Read the model definition and answer for the solid it produces. Units are mm, in the model's axes. Face numbers are marked on the shaded views. A direction names the side the tool comes from. Give positions to 0.01 mm unless a question says otherwise; leave off trailing zeros. Order: outer loops, then holes, each group sorted by start corner. A loop starts at its lowest first (then second) coordinate and runs counter-clockwise, first axis right, second up.
Item 1: A cutting plane is placed at C-C (x = -8.5). Write down the section's boundary in (y, z), plus the area to 3 significant figures.
Item 2: A cutting plane is placed at D-D (y = 1.5). Write down the section's boundary in (x, z).
Item 3: Find the intervals of material crossed by line 1 along Y through (x, z) = (-8.5, -0.5); line 2 along Y through (x, z) = (13, -0.25); line 3 along Z through (x, y) = (2, 7.5) (3 decimals), in increasing order.
Item 4: A cutting plane is placed at B-B (y = -8.95). Write down the section's boundary in (x, z) (3 decimals).
Item 5: A cutting plane is placed at A-A (x = 13). Write down the section's boundary in (y, z), plus the area to 3 significant figures.
Item 6: Which of the six approach directions +Z, -Z, +X, -X, +Y, -Y give full straight-line access (tool end or side, diameter ignored) to the marked faces 1 and 2?
Item 7: Given pin 1 Ø3 at (x, z) = (5, 2.5) entering from -Y; pin 2 Ø4 at (y, z) = (8, 4) entering from -X; pin 3 Ø2 at (x, z) = (18.5, 2) entering from -Y; pin 4 Ø1.4 at (x, y) = (4, -7) entering from +Z, each flat-ended and moving along its own axis, determine where each tip first touches the part or whether it passes through.
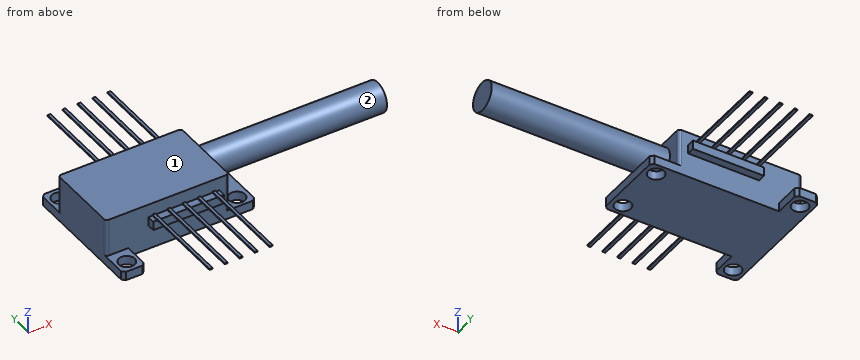
Autodesk Inventor part; units mm, degrees
ref_plane "Work Plane2" through (0, 0, 2.665) normal (0, 0, -1) x (-1, 0, 0)
ref_plane "YZ Plane" through (0, 0, 0) normal (1, 0, 0) x (0, 1, 0)
ref_plane "XZ Plane" through (0, 0, 0) normal (0, 1, 0) x (-1, 0, 0)
sketch "Sketch1" plane through (0, 0, 0) normal (0, 0, 1) x (1, 0, 0)
  line L0 (-10.4, -6.35) -> (10.4, -6.35)
  line L1 (10.4, -6.35) -> (10.4, 6.35)
  line L2 (10.4, 6.35) -> (-10.4, 6.35)
  line L3 (-10.4, 6.35) -> (-10.4, -6.35)
  line L4 (-10.4, -6.35) -> (10.4, 6.35) construction
  line L5 (10.4, -6.35) -> (-10.4, 6.35) construction
  point P0 (0, 0)
  dimension "d0" = 12.7
  dimension "d1" = 20.8
extrude "Extrusion1" add sketch "Sketch1" along normal blind 6.4
sketch "Sketch4" plane through (0, 0, 0) normal (0, 0, -1) x (-1, 0, 0)
  line L0 (10.4, -10.95) -> (6.6, -10.95)
  line L1 (-15, -6.35) -> (-15, 0)
  line L2 (-15, 0) -> (10.4, 0)
  line L3 (10.4, 0) -> (10.4, -10.95)
  line L4 (10.4, 6.35) -> (10.4, -6.35)
  line L5 (-15, -6.35) -> (6.6, -6.35)
  line L6 (6.6, -6.35) -> (6.6, -10.95)
  line L7 (10.4, -6.35) -> (-10.4, -6.35)
  point P0 (0, 0)
  dimension "d18" = 10.95
  dimension "d20" = 25.4
  dimension "d21" = 3.8
extrude "Extrusion4" add sketch "Sketch4" along normal blind 1.5
sketch "Sketch5" plane through (0, 0, -1.5) normal (0, 0, -1) x (-1, 0, 0)
  circle A0 centre (8.5, -8.95) radius 1.35
  circle A1 centre (-13, -4.45) radius 1.35
  line L0 (6.6, -10.95) -> (10.4, -10.95)
  line L1 (10.4, 0) -> (-15, 0)
  line L2 (10.4, -10.95) -> (10.4, 0)
  line L3 (-15, 0) -> (-15, -6.35)
  line L4 (-15, -6.35) -> (6.6, -6.35)
  point P0 (0, 0)
  dimension "d24" = 2.7
  dimension "d26" = 8.95
  dimension "d28" = 1.9
  dimension "d29" = 2
  dimension "d31" = 4.45
extrude "Extrusion5" cut sketch "Sketch5" against normal through all
chamfer "Chamfer2" distance 0.5 angle 45 3 edges at (-10.4, -10.95, -0.75) (-6.6, -10.95, -0.75) (15, -6.35, -0.75)
mirror "Mirror3" about plane through (0, 0, 0) normal (0, 1, 0) of "Extrusion4", "Extrusion5", "Chamfer2"
fillet "Fillet1" radius 0.5 4 edges at (10.4, -6.35, 3.2) (-10.4, -6.35, 3.2) (-10.4, 6.35, 3.2) (10.4, 6.35, 3.2)
ref_plane "Work Plane2" through (0, 0, 2.665) normal (0, 0, -1) x (-1, 0, 0)
sketch "Sketch6" plane through (0, 0, 2.665) normal (0, 0, -1) x (-1, 0, 0)
  line L0 (-9.9, 6.35) -> (9.9, 6.35)
  line L1 (-8.8, 6.35) -> (3.2, 6.35)
  line L2 (3.2, 6.35) -> (3.2, 7.65)
  line L3 (3.2, 7.65) -> (-8.8, 7.65)
  line L4 (-8.8, 7.65) -> (-8.8, 6.35)
  line L5 (-10.4, -5.85) -> (-10.4, 5.85)
  point P0 (0, 0)
  dimension "d39" = 1.3
  dimension "d40" = 12
  dimension "d41" = 1.6
extrude "Extrusion6" add sketch "Sketch6" against normal blind 1.5
sketch "Sketch7" plane through (0, 0, 4.165) normal (0, 0, 1) x (1, 0, 0)
  line L0 (8.8, 6.35) -> (-3.2, 6.35)
  line L1 (8.12, 6.35) -> (7.62, 6.35)
  line L2 (7.62, 6.35) -> (7.62, 21.65)
  line L3 (7.62, 21.65) -> (8.12, 21.65)
  line L4 (8.12, 21.65) -> (8.12, 6.35)
  line L5 (-15.48, 0) -> (20.08, 0)
  line L6 (7.87, 6.35) -> (7.87, 21.65) construction
  line L7 (10.4, -5.85) -> (10.4, 5.85)
  point P0 (0, 0)
  dimension "d46" = 21.65
  dimension "d47" = 2.53
  dimension "d48" = 0.5
extrude "Extrusion7" add sketch "Sketch7" along normal blind 0.2
pattern_linear "Rectangular Pattern1" count 5 spacing 2.54 along (-1, 0, 0) of "Extrusion7"
mirror "Mirror4" about plane through (0, 0, 0) normal (0, 1, 0) of "Extrusion6", "Extrusion7", "Rectangular Pattern1"
sketch "Sketch8" plane through (-10.4, -10.45, -1.5) normal (-1, 0, 0) x (0, 0, 1)
  line L0 (0, 0) -> (0, 20.9)
  line L1 (1.5, 4.1) -> (7.9, 4.1)
  point P0 (1.5, 10.45)
  point P1 (4.8, 8.6)
  dimension "d54" = 4.8
  dimension "d55" = 4.5
sketch "Sketch9" plane through (10.4, -5.85, 6.4) normal (1, 0, 0) x (0, 0, -1)
  line L0 (7.9, 0) -> (7.9, 11.7)
  line L1 (6.4, 12.2) -> (0, 12.2)
  circle A0 centre (3.2, 7.35) radius 2.5
  point P0 (6.4, 5.85)
  dimension "d56" = 4.7
  dimension "d57" = 4.85
  dimension "d58" = 5
extrude "fibre_connect" add sketch "Sketch9" along normal blind 30.15
ref_plane "Work Plane1" through (0, 0, 0) normal (0, 1, 0) x (-1, 0, 0)
ref_plane "Work Plane3" through (0, 0, 0) normal (0, 1, 0) x (-1, 0, 0)
properties part number "gainchip"
Response values:
1. outline: (-10.95, -1.5) - (-10.3, -1.5) - (-10.3, 0) - (-10.95, 0) - close; (-7.6, -1.5) - (7.6, -1.5) - (7.6, 0) - (6.35, 0) - (6.35, 6.4) - (-6.35, 6.4) - (-6.35, 0) - (-7.6, 0) - close; (10.3, -1.5) - (10.95, -1.5) - (10.95, 0) - (10.3, 0) - close
1. area: 106 mm2
2. outline: (-10.4, -1.5) - (15, -1.5) - (15, 0) - (10.4, 0) - (10.4, 0.7) - (40.55, 0.7) - (40.55, 5.7) - (10.4, 5.7) - (10.4, 6.4) - (-10.4, 6.4) - close
3. line 1: y = -10.95 to -10.3, -7.6 to 7.6, 10.3 to 10.95
3. line 2: y = -6.35 to -5.8, -3.1 to 3.1, 5.8 to 6.35
3. line 3: z = 2.665 to 4.165
4. outline: (-10.4, -1.5) - (-9.85, -1.5) - (-9.85, 0) - (-10.4, 0) - close; (-7.15, -1.5) - (-6.6, -1.5) - (-6.6, 0) - (-7.15, 0) - close; (-2.54, 4.165) - (-2.04, 4.165) - (-2.04, 4.365) - (-2.54, 4.365) - close; (0, 4.165) - (0.5, 4.165) - (0.5, 4.365) - (0, 4.365) - close; (2.54, 4.165) - (3.04, 4.165) - (3.04, 4.365) - (2.54, 4.365) - close; (5.08, 4.165) - (5.58, 4.165) - (5.58, 4.365) - (5.08, 4.365) - close; (7.62, 4.165) - (8.12, 4.165) - (8.12, 4.365) - (7.62, 4.365) - close
5. outline: (-6.35, -1.5) - (-5.8, -1.5) - (-5.8, 0) - (-6.35, 0) - close; (-3.1, -1.5) - (3.1, -1.5) - (3.1, 0) - (-3.1, 0) - close; circle Ø5 at (1.5, 3.2); (5.8, -1.5) - (6.35, -1.5) - (6.35, 0) - (5.8, 0) - close
5. area: 30.6 mm2
6. face 1: +Z, +X, -X, +Y, -Y
6. face 2: +X
7. pin 1: stops at y = -7.65
7. pin 2: stops at x = -10.38
7. pin 3: stops at y = -0.99
7. pin 4: stops at z = 6.4
